```python
from build123d import *

# Parameters (mm, degrees)
SKETCH_1_R          = 1.5
EXTRUDE_1_DEPTH     = 25
SKETCH_2_R          = 2.75
EXTRUDE_2_DEPTH     = 2.93
CUT_EXTRUDE_1_DEPTH = 1.3


with BuildPart() as part:
    # 草图1 → 凸台-拉伸1 (new body)
    with BuildSketch(Plane(origin=(0, 0, 0), x_dir=(1, 0, 0), z_dir=(0, 1, 0))):
        Circle(SKETCH_1_R)
    extrude(amount=EXTRUDE_1_DEPTH)

    # 草图2 → 凸台-拉伸2 (add)
    with BuildSketch(Plane(origin=(0, 25, 0), x_dir=(1, 0, 0), z_dir=(0, 1, 0))):
        Circle(SKETCH_2_R)
    extrude(amount=EXTRUDE_2_DEPTH)

    # 草图3 → 切除-拉伸1 (cut)
    with BuildSketch(Plane(origin=(0, 27.93, 0), x_dir=(1, 0, 0), z_dir=(0, 1, 0))):
        Polygon((1.024005842, -1.017224346), (1.392945046, 0.378202899), (0.368939204, 1.395427245), (-1.024005842, 1.017224346), (-1.392945046, -0.378202899), (-0.368939204, -1.395427245), align=None)
    extrude(amount=-CUT_EXTRUDE_1_DEPTH, mode=Mode.SUBTRACT)


solid = part.part
```
Model file for the job. Use its own axes, mm. A direction names the side the tool comes from. Coordinates: 2 decimals unless noted, no trailing zeros. Order: outer loops, then holes, each group sorted by start corner. A loop starts at its lowest first (then second) coordinate and runs counter-clockwise, first axis right, second up. Notation, with made-up numbers: (19.25, 22.5) -> (32.25, 22.5) arc R20 cw to (32.25, 50.5) -> close; hole circle Ø11 at (-6, 73). An arc over 180 degrees is marked (long way). Answer as a JSON object with one key per item and string values. Group by question number.
1) Which spindle directions (+Z, -Z, +X, -X, +Y, -Y) get a long thin tool onto all of the face, cutting with end or side? Do faces 1 (the face through (-0.89, 27.29, 0.88)), 2 (the face through (-0.596, 26.444, 2.685)), 3 (the face through (1.2, 25, 1.2)). Say none if no direction does.
2) Drill centre lines: L1, parallel to Y at x = -0.6, z = -1.85; L2, parallel to Z at x = -0.1, y = 8.5; L3, parallel to Y at x = 0.75, z = -0.35. Where is each one in solid material? Low to high.
3) Cut at B-B, the plane z = 0. Write the cut outline in (x, y).
4) Cut at A-A, the plane x = 0. Write the cut outline in (y, z).
5) Flat gauge pin, fed straight in: pin 1 (1.5 mm diameter, centred on y = 23, z = 0, fed in from -X). Where does the tip first touch, or does it go through?
6) Cut at D-D, the plane z = -1.95. Write the cut outline in (x, y).
7) Pull direction Z, two halves, no side cores. Call faces 4 (the face through (-0.32, 27.29, -1.21)), 5 (the face through (-1.5, 12.32, -0.07)), 6 (the face through (0, 0, 0)), 7 (the face through (-1.206, 27.289, -0.329)): +Z half, -Z half, draft (parallel to the pull), parting line (faces both ways), or undercut.
8) Cut at C-C, the plane y = 21.25. Write the cut outline in (x, z), then the cut area to 3 significant figures.
Check values:
{
 "1": {"face 1": "+Y", "face 2": "+Y, -Y", "face 3": "-Y"},
 "2": {"L1": "y = 25 to 27.93", "L2": "z = -1.5 to 1.5", "L3": "y = 0 to 26.63"},
 "3": {"outline": "(-2.75, 25) -> (-1.5, 25) -> (-1.5, 0) -> (1.5, 0) -> (1.5, 25) -> (2.75, 25) -> (2.75, 27.93) -> (1.29, 27.93) -> (1.29, 26.63) -> (-1.29, 26.63) -> (-1.29, 27.93) -> (-2.75, 27.93) -> close"},
 "4": {"outline": "(0, -1.5) -> (25, -1.5) -> (25, -2.75) -> (27.93, -2.75) -> (27.93, -1.3) -> (26.63, -1.3) -> (26.63, 1.3) -> (27.93, 1.3) -> (27.93, 2.75) -> (25, 2.75) -> (25, 1.5) -> (0, 1.5) -> close"},
 "5": {"pin 1": "stops at x = -1.5"},
 "6": {"outline": "(-1.94, 25) -> (1.94, 25) -> (1.94, 27.93) -> (-1.94, 27.93) -> close"},
 "7": {"face 4": "undercut", "face 5": "parting line", "face 6": "draft", "face 7": "undercut"},
 "8": {"outline": "circle Ø3 at (0, 0)", "area": "7.07 mm²"}
}
